from build123d import *

# Parameters (mm, degrees)
CROQUIS1_R              = 16
SALIENTE_EXTRUIR1_DEPTH = 5
CROQUIS2_R              = 1.75
CORTAR_EXTRUIR1_DEPTH   = 24.173260453
CORTAR_EXTRUIR2_DEPTH   = 3
SALIENTE_EXTRUIR2_START = 9
CROQUIS4_R              = 3
CROQUIS4_R_2            = 1.75
SALIENTE_EXTRUIR2_DEPTH = 9
CORTAR_EXTRUIR3_DEPTH   = 9
CORTAR_EXTRUIR7_DEPTH   = 9
CROQUIS7_W              = 11.2
CROQUIS7_H              = 4
CROQUIS7_W_2            = 9
CORTAR_EXTRUIR8_DEPTH   = 25.351591324
CROQUIS8_R              = 18.5
CROQUIS8_R_2            = 16
SALIENTE_EXTRUIR3_DEPTH = 2.5


with BuildPart() as part:
    # Croquis1 → Saliente-Extruir1 (new body)
    with BuildSketch(Plane.XY):
        Circle(CROQUIS1_R)
    extrude(amount=SALIENTE_EXTRUIR1_DEPTH)

    # Croquis2 → Cortar-Extruir1 (cut, through all)
    with BuildSketch(Plane.XY.offset(5)):
        with Locations((-8.025, 8.025)):
            Circle(CROQUIS2_R)
        with Locations((8.025, 8.025)):
            Circle(CROQUIS2_R)
        with Locations((8.025, -8.025)):
            Circle(CROQUIS2_R)
        with Locations((-8.025, -8.025)):
            Circle(CROQUIS2_R)
    extrude(amount=-CORTAR_EXTRUIR1_DEPTH, mode=Mode.SUBTRACT)

    # Croquis3 → Cortar-Extruir2 (cut)
    with BuildSketch(Plane(origin=(0, 0, 0), x_dir=(-1, 0, 0), z_dir=(0, 0, -1))):
        Polygon((-4.560898385, 8.025), (-6.292949192, 11.025), (-9.757050808, 11.025), (-11.489101615, 8.025), (-9.757050808, 5.025), (-6.292949192, 5.025), align=None)
        Polygon((6.292949192, 5.025), (4.560898385, 8.025), (6.292949192, 11.025), (9.757050808, 11.025), (11.489101615, 8.025), (9.757050808, 5.025), align=None)
        Polygon((9.757050808, -5.025), (6.292949192, -5.025), (4.560898385, -8.025), (6.292949192, -11.025), (9.757050808, -11.025), (11.489101615, -8.025), align=None)
        Polygon((-6.292949192, -5.025), (-4.560898385, -8.025), (-6.292949192, -11.025), (-9.757050808, -11.025), (-11.489101615, -8.025), (-9.757050808, -5.025), align=None)
    extrude(amount=-CORTAR_EXTRUIR2_DEPTH, mode=Mode.SUBTRACT)

    # Croquis4 → Saliente-Extruir2 (add)
    # profile 1 of 4: a face of its own
    with BuildSketch(Plane.XY.offset(5).offset(SALIENTE_EXTRUIR2_START)):
        with Locations((-8.025, 8.025)):
            Circle(CROQUIS4_R)
        with Locations((-8.025, 8.025)):
            Circle(CROQUIS4_R_2, mode=Mode.SUBTRACT)
    # profile 2 of 4: a face of its own
    with BuildSketch(Plane.XY.offset(5).offset(SALIENTE_EXTRUIR2_START)):
        with Locations((8.025, 8.025)):
            Circle(CROQUIS4_R)
        with Locations((8.025, 8.025)):
            Circle(CROQUIS4_R_2, mode=Mode.SUBTRACT)
    # profile 3 of 4: a face of its own
    with BuildSketch(Plane.XY.offset(5).offset(SALIENTE_EXTRUIR2_START)):
        with Locations((-8.025, -8.025)):
            Circle(CROQUIS4_R)
        with Locations((-8.025, -8.025)):
            Circle(CROQUIS4_R_2, mode=Mode.SUBTRACT)
    # profile 4 of 4: a face of its own
    with BuildSketch(Plane.XY.offset(5).offset(SALIENTE_EXTRUIR2_START)):
        with Locations((8.025, -8.025)):
            Circle(CROQUIS4_R)
        with Locations((8.025, -8.025)):
            Circle(CROQUIS4_R_2, mode=Mode.SUBTRACT)
    extrude(amount=-SALIENTE_EXTRUIR2_DEPTH)

    # Croquis5 → Cortar-Extruir3 (cut)
    with BuildSketch(Plane.XY.offset(14)):
        with BuildLine():
            Line((-5.025, 8.025), (-8.025, 5.025))
            ThreePointArc((-8.025, 5.025), (-5.903679656, 5.903679656), (-5.025, 8.025))
        make_face()
        with BuildLine():
            Line((5.025, 8.025), (8.025, 5.025))
            ThreePointArc((8.025, 5.025), (5.903679656, 5.903679656), (5.025, 8.025))
        make_face()
    extrude(amount=-CORTAR_EXTRUIR3_DEPTH, mode=Mode.SUBTRACT)

    # Croquis6 → Cortar-Extruir7 (cut)
    with BuildSketch(Plane.XY.offset(14)):
        with BuildLine():
            Line((-6.22430322, 6.82569678), (-5.025, 8.025))
            ThreePointArc((-5.025, 8.025), (-5.341523678, 9.366251218), (-6.22430322, 10.424477257))
            Line((-6.22430322, 10.424477257), (-6.22430322, 6.82569678))
        make_face()
        with BuildLine():
            Line((6.22430322, 10.424477257), (6.22430322, 6.82569678))
            Line((6.22430322, 6.82569678), (5.025, 8.025))
            ThreePointArc((5.025, 8.025), (5.341523678, 9.366251218), (6.22430322, 10.424477257))
        make_face()
    extrude(amount=-CORTAR_EXTRUIR7_DEPTH, mode=Mode.SUBTRACT)

    # Croquis7 → Cortar-Extruir8 (cut, through all)
    with BuildSketch(Plane.XY.offset(5)):
        with Locations((0, 6)):
            Rectangle(CROQUIS7_W, CROQUIS7_H)
        with Locations((0, -6)):
            Rectangle(CROQUIS7_W_2, CROQUIS7_H)
    extrude(amount=-CORTAR_EXTRUIR8_DEPTH, mode=Mode.SUBTRACT)

    # Croquis8 → Saliente-Extruir3 (add)
    with BuildSketch(Plane(origin=(0, 0, 0), x_dir=(-1, 0, 0), z_dir=(0, 0, -1))):
        Circle(CROQUIS8_R)
        Circle(CROQUIS8_R_2, mode=Mode.SUBTRACT)
    extrude(amount=-SALIENTE_EXTRUIR3_DEPTH)


solid = part.part
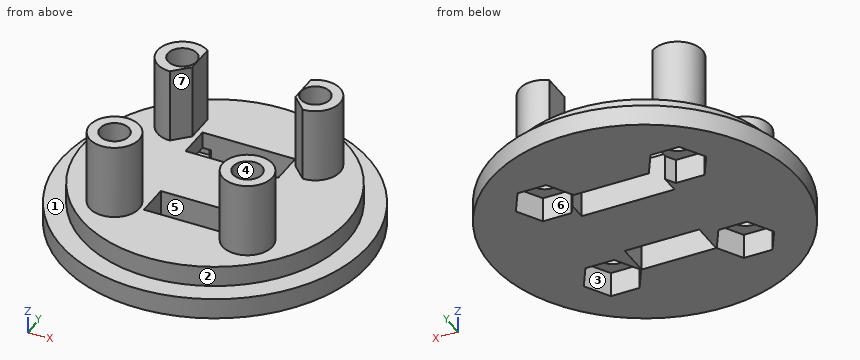
The listing builds one solid part. Answer for the finished solid, in the listing's coordinates (mm). Face numbers are marked on the shaded views. A direction names the side the tool comes from. Give positions to 0.01 mm unless a question says otherwise; leave off trailing zeros. Loops run counter-clockwise (first coordinate to the right, second up) from the corner with the lowest first, then second, coordinate; pieces in that order, holes last.
Item 1: A tool of negligible diameter and unlimited length cuts with its end or side. For the marked faces 5, 6 and 7, from which of +Z, -Z, +X, -X, +Y, -Y can it reach the whole face along a straight path? Write none if from no direction.
Derived:
face 5: +Z, -Z
face 6: -Z
face 7: +Z
Item 2: A cutting plane is placed at D-D (x = -14). Give the vertices of the cut face in (y, z).
Derived:
outline: (-12.09, 0) - (12.09, 0) - (12.09, 2.5) - (7.75, 2.5) - (7.75, 5) - (-7.75, 5) - (-7.75, 2.5) - (-12.09, 2.5) - close
Item 3: Find the intervals of material crossed by line 1 along X through (y, z) = (8.5, 1.25); line 2 along Y through (x, z) = (7.5, 11); line 3 along X through (y, z) = (6.5, 12.75), in increasing order.
Derived:
line 1: x = -16.43 to -11.21, -4.84 to 4.84, 11.21 to 16.43
line 2: y = -10.98 to -9.69, -6.36 to -5.07, 5.55 to 6.36, 9.69 to 10.98
line 3: x = -10.61 to -8.88, -7.17 to -6.55, 6.55 to 7.17, 8.88 to 10.61
Item 4: Each of these flat-tipped pins is pushed along its axis until it touches: pin 1 Ø1 at (y, z) = (-3.5, 4) entering from +X; pin 2 Ø2 at (x, y) = (-8.025, 8.025) entering from -Z; pin 3 Ø2.5 at (x, z) = (7.5, 2) entering from -Y; pin 4 Ø2.5 at (x, z) = (-1, 2) entering from -Y. Where does it stop, or does it pass through?
Derived:
pin 1: stops at x = 15.72
pin 2: passes through
pin 3: stops at y = -17.41
pin 4: stops at y = -18.5
Item 5: A cutting plane is placed at B-B (x = 0). Give the vertices of the cut face in (y, z).
Derived:
outline: (-18.5, 0) - (-8, 0) - (-8, 5) - (-16, 5) - (-16, 2.5) - (-18.5, 2.5) - close; (-4, 0) - (4, 0) - (4, 5) - (-4, 5) - close; (8, 0) - (18.5, 0) - (18.5, 2.5) - (16, 2.5) - (16, 5) - (8, 5) - close
Item 6: A cutting plane is placed at A-A (z = 7.25). Give the vertices of the cut face in (x, y) (3 decimals), then the cut area to 3 significant figures.
Derived:
outline: circle Ø6 at (-8.025, -8.025); (-8.025, 5.025) - (-6.224, 6.826) - (-6.224, 10.424) arc R3 ccw (long way) to start; circle Ø6 at (8.025, -8.025); (6.224, 6.826) - (8.025, 5.025) arc R3 ccw (long way) to (6.224, 10.424) - close; hole circle Ø3.5 at (-8.025, -8.025); hole circle Ø3.5 at (-8.025, 8.025); hole circle Ø3.5 at (8.025, -8.025); hole circle Ø3.5 at (8.025, 8.025)
area: 64.0 mm2
Item 7: Determine the mould class of the marked faces 1, 2, 3 and 4 for opening direction Y: +Y half, -Y half, draft (parallel to the pull), parting line (faces both ways), or undercut.
Derived:
face 1: draft
face 2: parting line
face 3: undercut
face 4: undercut
Item 8: A cutting plane is placed at C-C (y = 0). Give the vertices of the cut face in (x, z).
Derived:
outline: (-18.5, 0) - (18.5, 0) - (18.5, 2.5) - (16, 2.5) - (16, 5) - (-16, 5) - (-16, 2.5) - (-18.5, 2.5) - close
